```python
from build123d import *

# Parameters (mm, degrees)
CROQUIS1_W                = 12
CROQUIS1_H                = 15
CROQUIS1_W_2              = 8
CROQUIS1_H_2              = 11
SALIENTE_EXTRUIR1_DEPTH   = 159.5
CROQUIS2_R                = 2.5
SALIENTE_EXTRUIR2_DEPTH   = 2
SIMETR_A2_COPY_1_SKETCH_R = 2.5
SIMETR_A2_COPY_1_DEPTH    = 2
SKETCH1_W                 = 159.5
SKETCH1_H                 = 34.305734292
CUT_EXTRUDE1_DEPTH        = 3
CUT_EXTRUDE1_DEPTH_BACK   = 15
SKETCH5_R                 = 2.5
CUT_EXTRUDE2_DEPTH        = 15
SKETCH6_W                 = 5
SKETCH6_H                 = 15
CUT_EXTRUDE3_DEPTH        = 3
CUT_EXTRUDE3_DEPTH_BACK   = 15


with BuildPart() as part:
    # Croquis1 → Saliente-Extruir1 (new body, symmetric)
    with BuildSketch(Plane.XY):
        Rectangle(CROQUIS1_W, CROQUIS1_H)
        Rectangle(CROQUIS1_W_2, CROQUIS1_H_2, mode=Mode.SUBTRACT)
    extrude(amount=SALIENTE_EXTRUIR1_DEPTH, both=True)

    # Croquis2 → Saliente-Extruir2 (add)
    with BuildSketch(Plane(origin=(6, 0, 0), x_dir=(0, 0, -1), z_dir=(1, 0, 0))):
        with BuildLine():
            Line((-145, -14.5), (-145, -0.5))
            Line((-145, -0.5), (-135, -0.5))
            Line((-135, -0.5), (-135, -14.5))
            ThreePointArc((-135, -14.5), (-140, -19.5), (-145, -14.5))
        make_face()
        with Locations((-140, -14.5)):
            Circle(CROQUIS2_R, mode=Mode.SUBTRACT)
    saliente_extruir2 = extrude(amount=SALIENTE_EXTRUIR2_DEPTH)

    # Simetría1: Saliente-Extruir2 across plane
    add(saliente_extruir2.mirror(Plane(origin=(0, 0, 0), x_dir=(0, 0, 1), z_dir=(1, 0, 0))))

    # Simetría2: Saliente-Extruir2 across plane
    add(saliente_extruir2.mirror(Plane.XY))

    # Simetría2 copy 1 sketch → Simetría2 copy 1 (add)
    with BuildSketch(Plane.ZY.offset(6)):
        with BuildLine():
            Line((-145, -14.5), (-145, -0.5))
            Line((-145, -0.5), (-135, -0.5))
            Line((-135, -0.5), (-135, -14.5))
            ThreePointArc((-135, -14.5), (-140, -19.5), (-145, -14.5))
        make_face()
        with Locations((-140, -14.5)):
            Circle(SIMETR_A2_COPY_1_SKETCH_R, mode=Mode.SUBTRACT)
    extrude(amount=SIMETR_A2_COPY_1_DEPTH)

    # Sketch1 → Cut-Extrude1 (cut, two sides)
    with BuildSketch(Plane(origin=(6, 0, 0), x_dir=(0, 0, -1), z_dir=(1, 0, 0))) as cut_extrude1_sk:
        with Locations((-79.75, -9.652867146)):
            Rectangle(SKETCH1_W, SKETCH1_H)
    extrude(amount=CUT_EXTRUDE1_DEPTH, mode=Mode.SUBTRACT)
    extrude(cut_extrude1_sk.sketch, amount=-CUT_EXTRUDE1_DEPTH_BACK, mode=Mode.SUBTRACT)

    # Sketch5 → Cut-Extrude2 (cut, through all)
    with BuildSketch(Plane.ZY.offset(6)):
        with Locations((-9, 1)):
            Circle(SKETCH5_R)
    extrude(amount=-CUT_EXTRUDE2_DEPTH, mode=Mode.SUBTRACT)

    # Sketch6 → Cut-Extrude3 (cut, two sides)
    with BuildSketch(Plane.ZY.offset(6)) as cut_extrude3_sk:
        with Locations((-157, 0)):
            Rectangle(SKETCH6_W, SKETCH6_H)
    extrude(amount=CUT_EXTRUDE3_DEPTH, mode=Mode.SUBTRACT)
    extrude(cut_extrude3_sk.sketch, amount=-CUT_EXTRUDE3_DEPTH_BACK, mode=Mode.SUBTRACT)


solid = part.part
```
Check sheet for the modelled part. Datum: model origin and axes. Units: mm. A direction names the side the tool comes from. Coordinates: 2 decimals unless noted, no trailing zeros. Loops run counter-clockwise (first coordinate to the right, second up) from the corner with the lowest first, then second, coordinate; pieces in that order, holes last.
1) Sectioned sample at A-A (z = -140). Record the boundary of the cut face in (x, y), and give its area (3 significant figures).
2) Material ranges on probe 1 along Y at (x, z) = (1.5, -37.5); probe 2 along Y at (x, z) = (-7.6, -140); probe 3 along X at (y, z) = (-3, -108), recorded low to high.
3) Sectioned sample at D-D (z = -9). Record the boundary of the cut face in (x, y).
4) Gauge pin test, flat ends, axial feed: pin 1 (3.5 mm diameter, centred on y = -2, z = -97.5, fed in from +X); pin 2 (3 mm diameter, centred on x = 2.5, z = -136.5, fed in from -Y); pin 3 (6 mm diameter, centred on y = 1.5, z = -60, fed in from -X). Record the tip position at first contact, or that the pin passes through.
5) Sectioned sample at C-C (y = 1). Record the boundary of the cut face in (x, z).
6) Access from +Z, -Z, +X, -X, +Y, -Y to the whole of each face (thin tool, end or side, straight path). Record for faces 4 (the face through (-4, 0, -76)), 5 (the face through (6.99, -15.46, -137.69)), 6 (the face through (6, -12, -139)).
7) Sectioned sample at B-B (x = 2.5). Record the boundary of the cut face in (y, z).
8) Release check for a two-part mould opening along Z. For faces 1 (the face through (4.99, 2.69, -10.84)), 2 (the face through (4, 0, -76)), 3 (the face through (7, -19.5, -139.9)) record: released by +Z, released by -Z, zero draft, split by the parting line, or undercut.
Check sheet entries:
1. outline: (-8, -19.5) - (-6, -19.5) - (-6, -17) - (-8, -17) - close; (-8, -12) - (-6, -12) - (-6, -7.5) - (6, -7.5) - (6, -12) - (8, -12) - (8, -0.5) - (6, -0.5) - (6, 7.5) - (-6, 7.5) - (-6, -0.5) - (-8, -0.5) - close; (6, -19.5) - (8, -19.5) - (8, -17) - (6, -17) - close; hole (-4, -5.5) - (4, -5.5) - (4, 5.5) - (-4, 5.5) - close
1. area: 148 mm2
2. probe 1: y = -7.5 to -5.5, 5.5 to 7.5
2. probe 2: y = -19.5 to -17, -12 to -0.5
2. probe 3: x = -6 to -4, 4 to 6
3. outline: (-6, -7.5) - (6, -7.5) - (6, -1.5) - (4, -1.5) - (4, -5.5) - (-4, -5.5) - (-4, -1.5) - (-6, -1.5) - close; (-6, 3.5) - (-4, 3.5) - (-4, 5.5) - (4, 5.5) - (4, 3.5) - (6, 3.5) - (6, 7.5) - (-6, 7.5) - close
4. pin 1: stops at x = 6
4. pin 2: stops at y = -7.5
4. pin 3: stops at x = -6
5. outline: (-6, -154.5) - (-4, -154.5) - (-4, -11.5) - (-6, -11.5) - close; (-6, -6.5) - (-4, -6.5) - (-4, 0) - (-6, 0) - close; (4, -154.5) - (6, -154.5) - (6, -11.5) - (4, -11.5) - close; (4, -6.5) - (6, -6.5) - (6, 0) - (4, 0) - close
6. face 4: +Z, -Z
6. face 5: +X, -X
6. face 6: +Z, -Z, -Y
7. outline: (-7.5, -154.5) - (-5.5, -154.5) - (-5.5, 0) - (-7.5, 0) - close; (5.5, -154.5) - (7.5, -154.5) - (7.5, 0) - (5.5, 0) - close
8. face 1: undercut
8. face 2: zero draft
8. face 3: split by the parting line
